```python
from build123d import *

# Parameters (mm, degrees)
SKETCH_1_W          = 50
SKETCH_1_H          = 52
EXTRUDE_1_DEPTH     = 3
SKETCH_2_W          = 50
SKETCH_2_H          = 3
EXTRUDE_2_DEPTH     = 54
SKETCH_3_R          = 11
SKETCH_3_R_2        = 2
SKETCH_3_R_3        = 1.75
CUT_EXTRUDE_1_DEPTH = 68.453687816
CHAMFER_1_SIZE      = 5
CHAMFER_2_SIZE      = 5
CUT_EXTRUDE_2_DEPTH = 80.025312401
EXTRUDE_START       = -50
EXTRUDE_3_DEPTH     = 50
CUT_EXTRUDE_START   = -3
CUT_EXTRUDE_3_DEPTH = 44
FILLET_1_R          = 5


with BuildPart() as part:
    # 草圖1 → 填料-伸長1 (new body)
    with BuildSketch(Plane.XY):
        Rectangle(SKETCH_1_W, SKETCH_1_H)
    extrude(amount=EXTRUDE_1_DEPTH)

    # 草圖2 → 填料-伸長2 (add)
    with BuildSketch(Plane(origin=(0, 0, 0), x_dir=(-1, 0, 0), z_dir=(0, 0, -1))):
        with Locations((0, -24.5)):
            Rectangle(SKETCH_2_W, SKETCH_2_H)
    extrude(amount=EXTRUDE_2_DEPTH)

    # 草圖3 → 除料-伸長1 (cut, through all)
    with BuildSketch(Plane.XY.offset(3)):
        with Locations((0, 5)):
            Circle(SKETCH_3_R)
        with Locations((14.5, 5)):
            Circle(SKETCH_3_R_2)
        with Locations((-14.5, 5)):
            Circle(SKETCH_3_R_2)
        with Locations((-15.5, -10.5)):
            Circle(SKETCH_3_R_3)
        with Locations((-15.5, 20.5)):
            Circle(SKETCH_3_R_3)
        with Locations((15.5, 20.5)):
            Circle(SKETCH_3_R_3)
        with Locations((15.5, -10.5)):
            Circle(SKETCH_3_R_3)
    extrude(amount=-CUT_EXTRUDE_1_DEPTH, mode=Mode.SUBTRACT)

    # 導角1
    chamfer_1_edges = [part.edges().sort_by_distance(p)[0] for p in [
        (-25, 26, 1.5),
        (25, 26, 1.5),
    ]]
    chamfer(chamfer_1_edges, length=CHAMFER_1_SIZE)

    # 導角2
    chamfer_2_edges = [part.edges().sort_by_distance(p)[0] for p in [
        (25, -24.5, -54),
        (-25, -24.5, -54),
    ]]
    chamfer(chamfer_2_edges, length=CHAMFER_2_SIZE)

    # 草圖4 → 除料-伸長2 (cut, through all)
    with BuildSketch(Plane.XZ.offset(26)):
        with BuildLine():
            Line((13, -43), (13, -13))
            ThreePointArc((13, -13), (15, -11), (17, -13))
            Line((17, -13), (17, -43))
            ThreePointArc((17, -43), (15, -45), (13, -43))
        make_face()
        with BuildLine():
            Line((-13, -43), (-13, -13))
            ThreePointArc((-13, -13), (-15, -11), (-17, -13))
            Line((-17, -13), (-17, -43))
            ThreePointArc((-17, -43), (-15, -45), (-13, -43))
        make_face()
    extrude(amount=-CUT_EXTRUDE_2_DEPTH, mode=Mode.SUBTRACT)

    # 草圖5 → 填料-伸長3 (add)
    with BuildSketch(Plane(origin=(25, 0, 0), x_dir=(0, 0, -1), z_dir=(1, 0, 0)).offset(EXTRUDE_START)):
        Polygon((0, -23), (0, -3), (14, -23), align=None)
    extrude(amount=EXTRUDE_3_DEPTH)

    # 草圖6 → 除料-伸長3 (cut)
    with BuildSketch(Plane(origin=(25, 0, 0), x_dir=(0, 0, -1), z_dir=(1, 0, 0)).offset(CUT_EXTRUDE_START)):
        Polygon((0, -3), (14, -23), (0, -23), align=None)
    extrude(amount=-CUT_EXTRUDE_3_DEPTH, mode=Mode.SUBTRACT)

    # 圓角1
    fillet_1_edges = [part.edges().sort_by_distance(p)[0] for p in [
        (0, -26, 3),
    ]]
    fillet(fillet_1_edges, radius=FILLET_1_R)


solid = part.part
```
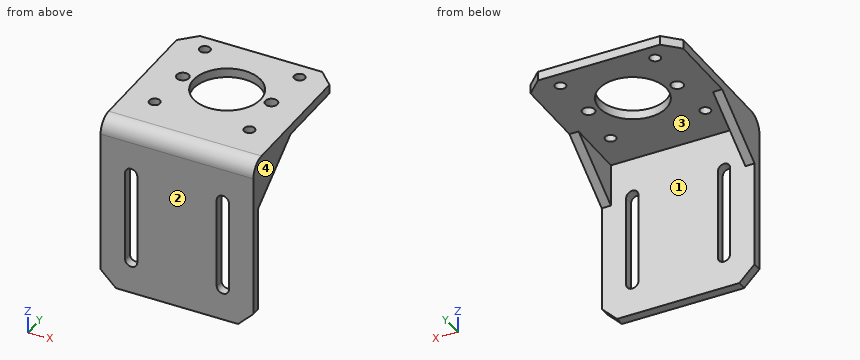
Design review of the part built by this model. Coordinates are the model's own, in mm. Face numbers are marked on the shaded views. Give positions to 0.01 mm unless a question says otherwise; leave off trailing zeros. Loops run counter-clockwise (first coordinate to the right, second up) from the corner with the lowest first, then second, coordinate; pieces in that order, holes last. Notation, with made-up numbers: (34.5, -34.75) -> (66.5, -34.75) arc R21 cw to (66.5, -29.75) -> close; hole circle Ø11 at (61, 64.25). An arc over 180 degrees is marked (long way). Write each question's results on one line, items separated by ' | '.
Q1. Wall thickness on L1, parallel to X at y = 22, z = 1; L2, parallel to Y at x = -14.5, z = 2.4; L3, parallel to Y at x = -5, z = -32: over which ranges is each line inside the solid? List them lowest first.
Reply:
L1: x = -24 to -16.4, -14.6 to 14.6, 16.4 to 24 | L2: y = -23.37 to -11.94, -9.06 to 3, 7 to 19.06, 21.94 to 26 | L3: y = -26 to -23
Q2. Take a section at A-A, the plane y = 5. Write out the cut boundary in (x, z).
Reply:
outline: (-25, 0) -> (-16.5, 0) -> (-16.5, 3) -> (-25, 3) -> close; (-12.5, 0) -> (-11, 0) -> (-11, 3) -> (-12.5, 3) -> close; (11, 0) -> (12.5, 0) -> (12.5, 3) -> (11, 3) -> close; (16.5, 0) -> (25, 0) -> (25, 3) -> (16.5, 3) -> close
Q3. Take a section at B-B, the plane z = -19.5. Write out the cut boundary in (x, y), plus the area to 3 significant figures.
Reply:
outline: (-25, -26) -> (-17, -26) -> (-17, -23) -> (-25, -23) -> close; (-13, -26) -> (13, -26) -> (13, -23) -> (-13, -23) -> close; (17, -26) -> (25, -26) -> (25, -23) -> (17, -23) -> close | area: 126 mm²
Q4. The part is to be moulded in two halves that separate along X. For the marked faces 1, 2, 3 and 4, say which applies: +X half, -X half, draft (parallel to the pull), parting line (faces both ways), or undercut.
Reply:
face 1: undercut | face 2: draft | face 3: undercut | face 4: +X half
Q5. Take a section at C-C, the plane x = 15.5. Write out the cut boundary in (y, z), plus the area to 3 significant figures.
Reply:
outline: (-26, -54) -> (-23, -54) -> (-23, -44.94) -> (-26, -44.94) -> close; (-26, -11.06) -> (-23, -11.06) -> (-23, 0) -> (-12.25, 0) -> (-12.25, 3) -> (-21, 3) arc R5 ccw to (-26, -2) -> close; (-8.75, 0) -> (3.27, 0) -> (3.27, 3) -> (-8.75, 3) -> close; (6.73, 0) -> (18.75, 0) -> (18.75, 3) -> (6.73, 3) -> close; (22.25, 0) -> (26, 0) -> (26, 3) -> (22.25, 3) -> close | area: 180 mm²
Q6. Take a section at D-D, the plane y = -19. Write out the cut boundary in (x, z), plus the area to 3 significant figures.
Reply:
outline: (-25, -11.2) -> (-22, -11.2) -> (-22, 0) -> (22, 0) -> (22, -11.2) -> (25, -11.2) -> (25, 3) -> (-25, 3) -> close | area: 217 mm²
Q7. For pin 1 Ø1 at (x, z) = (-11, -18) entering from +Y; pin 2 Ø4 at (x, y) = (15.5, 20.5) entering from -Z, all flat-tipped, find the tip position at first contact; note any pin that passes through.
Reply:
pin 1: stops at y = -23 | pin 2: stops at z = 0
